Geometry check sheet. Reference: drawing and pictorial views, mm from the part's lowest x, y, z. Round coordinates to 2 decimals unless told otherwise and drop trailing zeros. Write each loop counter-clockwise with the first axis right and the second up, starting at its lowest first coordinate (ties: lowest second). Pieces come first, ordered by that corner, then holes. Notation, with made-up numbers: M -32.5,-24.5 L 6.5,-24.5 A23 ccw 6.5,8.5 Z; hole C 62.25,56 d7. An arc over 180 degrees is marked long. Use a Markdown table: item, result. Add a question column.
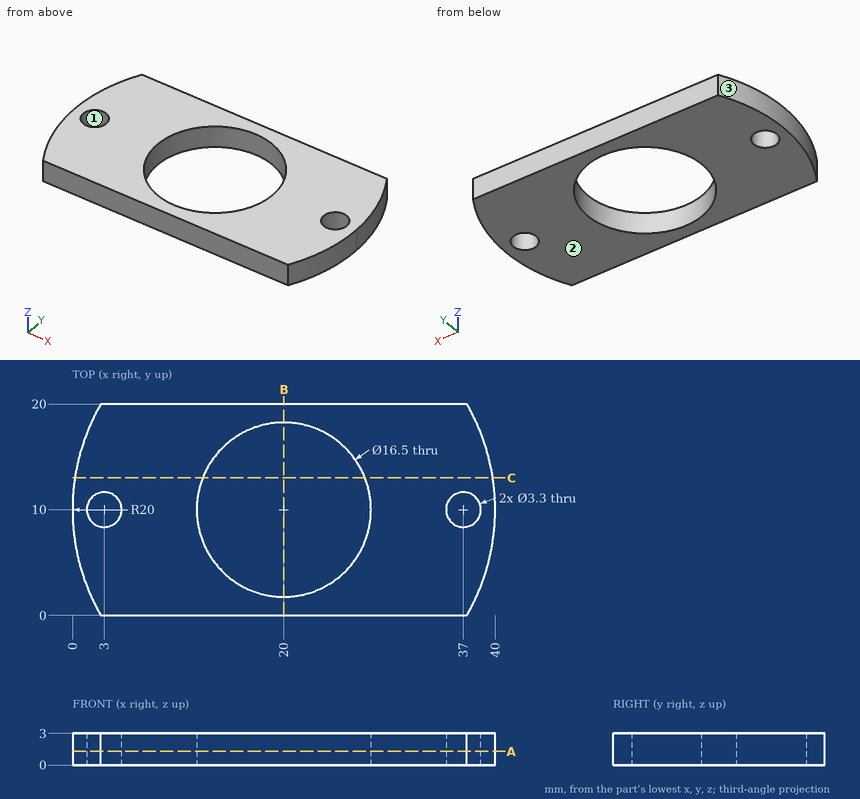
1. Scan lines: line 1 along Y through (x, z) = (3, 0.95); line 2 along Y through (x, z) = (20, 1.85); line 3 along X through (y, z) = (11.5, 1.1). Record each from-to range of solid material in increasing order. Write a range as from..to.
2. Cross-section at B-B on x = 20. Enter the section's corners in (y, z), plus the area to 3 significant figures.
3. Cross-section at A-A on z = 1.3. Enter the section's corners in (x, y).
4. Cross-section at C-C on y = 13. Enter the section's corners in (x, z), plus the area to 3 significant figures.
5. Release check for a two-part mould opening along Y. For the marked faces 1, 2 and 3 record: +Y half, -Y half, draft (parallel to the pull), parting line (faces both ways), or undercut.
Answer:
| question | item | result |
|---|---|---|
| 1 | line 1 | y = 0..8.35, 11.65..20 |
| 1 | line 2 | y = 0..1.75, 18.25..20 |
| 1 | line 3 | x = 0.06..2.31, 3.69..11.89, 28.11..36.31, 37.69..39.94 |
| 2 | outline | M 0,0 L 1.75,0 L 1.75,3 L 0,3 Z; M 18.25,0 L 20,0 L 20,3 L 18.25,3 Z |
| 2 | area | 10.5 mm^2 |
| 3 | outline | M 2.68,0 L 37.32,0 A20 ccw 37.32,20 L 2.68,20 A20 ccw Z; hole C 3,10 d3.3; hole C 20,10 d16.5; hole C 37,10 d3.3 |
| 4 | outline | M 0.23,0 L 12.31,0 L 12.31,3 L 0.23,3 Z; M 27.69,0 L 39.77,0 L 39.77,3 L 27.69,3 Z |
| 4 | area | 72.5 mm^2 |
| 5 | face 1 | undercut |
| 5 | face 2 | draft |
| 5 | face 3 | parting line |
